Read the model definition and answer for the solid it produces. Units are mm, in the model's axes. Face numbers are marked on the shaded views. A direction names the side the tool comes from. Coordinates: 2 decimals unless noted, no trailing zeros. Order: outer loops, then holes, each group sorted by start corner. A loop starts at its lowest first (then second) coordinate and runs counter-clockwise, first axis right, second up. Notation, with made-up numbers: (64, -34.5) -> (109, -34.5) arc R32 ccw to (109, -1.5) -> close; hole circle Ø11 at (-16.5, -32.75). An arc over 180 degrees is marked (long way). Answer as a JSON object with one key per item and string values. Group by question number.
1) Section C-C on y = 135 is taken. Determine the outline of the cut face in (x, z), and give its area (3 significant figures).
2) Section D-D on x = 12.5 is taken. Determine the outline of the cut face in (y, z).
3) Section A-A on y = 45 is taken. Determine the outline of the cut face in (x, z).
4) Consider L1, parallel to Y at x = 26.75, z = 0; L2, parallel to Y at x = 28.5, z = 0.5; L3, parallel to X at y = -1.5, z = -9. Determine where each line is inside the solid, lowest interval first.
5) Given pin 1 (4 mm diameter, centred on x = 23.5, z = -6, fed in from +Y); pin 2 (5 mm diameter, centred on x = 18.5, y = 40, fed in from -Z); pin 3 (3 mm diameter, centred on x = 23, z = 4.5, fed in from +Y), each flat-ended and moving along its own axis, determine where each tip first touches the part or whether it passes through.
6) Section B-B on x = 31 is taken. Determine the outline of the cut face in (y, z), and give its area (3 significant figures).
7) Determine the mould class of the marked faces 1, 2, 3 and 4 for opening direction Z: released by +Z, released by -Z, zero draft, split by the parting line, or undercut.
8) A tool of negligible diameter and unlimited length cuts with its end or side. For the marked faces 5, 6 and 7, from which of +Z, -Z, +X, -X, +Y, -Y can it reach the whole face along a straight path? Write none if from no direction.
from build123d import *

# Parameters (mm, degrees)
SKETCH1_R               = 2
BOSS_EXTRUDE1_DEPTH     = 33
CUT_EXTRUDE1_DEPTH      = 13.5
CUT_EXTRUDE2_DEPTH      = 16.5
SKETCH4_R               = 2
CUT_EXTRUDE3_DEPTH      = 5
CUT_EXTRUDE4_DEPTH      = 3
CUT_EXTRUDE5_DEPTH      = 151.15655797
CUT_EXTRUDE5_DEPTH_BACK = 151.15655797


with BuildPart() as part:
    # Sketch1 → Boss-Extrude1 (new body)
    with BuildSketch(Plane(origin=(0, 0, 0), x_dir=(0, 0, -1), z_dir=(1, 0, 0))):
        with BuildLine():
            ThreePointArc((-15.746923292, -2.834502924), (3.806207647, -15.54068156), (15.274538651, 4.763241437))
            ThreePointArc((15.274538651, 4.763241437), (4.169990688, 68.449264041), (9.766892503, 132.853418803))
            ThreePointArc((9.766892503, 132.853418803), (2.382772527, 144.71197174), (-9.651340082, 137.617562724))
            ThreePointArc((-9.651340082, 137.617562724), (-20.507516508, 67.730411775), (-15.746923292, -2.834502924))
        make_face()
        with Locations((0, 135)):
            Circle(SKETCH1_R, mode=Mode.SUBTRACT)
        Circle(SKETCH1_R, mode=Mode.SUBTRACT)
        with BuildLine():
            ThreePointArc((-12.675406771, 58.150621112), (-12.300365948, 46.179147672), (-11.058070356, 34.266400985))
            ThreePointArc((-11.058070356, 34.266400985), (-5.587650283, 30.149080215), (-1.470329513, 35.619500288))
            ThreePointArc((-1.470329513, 35.619500288), (-2.639739364, 46.833323654), (-2.992776465, 58.102428263))
            ThreePointArc((-2.992776465, 58.102428263), (-7.809995194, 62.967839841), (-12.675406771, 58.150621112))
        make_face(mode=Mode.SUBTRACT)
        with BuildLine():
            ThreePointArc((-10.574940666, 104.538451831), (-12.44695641, 91.799336957), (-12.717862815, 78.926260385))
            ThreePointArc((-12.717862815, 78.926260385), (-7.68030208, 74.289364014), (-3.04340571, 79.326924749))
            ThreePointArc((-3.04340571, 79.326924749), (-2.79792055, 90.992020929), (-1.101570529, 102.535726074))
            ThreePointArc((-1.101570529, 102.535726074), (-4.836892719, 108.273774021), (-10.574940666, 104.538451831))
        make_face(mode=Mode.SUBTRACT)
    extrude(amount=BOSS_EXTRUDE1_DEPTH)

    # Sketch2 → Cut-Extrude1 (cut)
    with BuildSketch(Plane.ZY.offset(-8.25)):
        with BuildLine():
            ThreePointArc((9.651340082, 137.617562724), (-2.382772527, 144.71197174), (-9.766892503, 132.853418803))
            ThreePointArc((-9.766892503, 132.853418803), (-8.074404211, 124.471332441), (-6.669573364, 116.036266424))
            ThreePointArc((-6.669573364, 116.036266424), (4.209591857, 115.639688485), (13.684813674, 121.000069207))
            ThreePointArc((13.684813674, 121.000069207), (11.779096359, 129.335763119), (9.651340082, 137.617562724))
        make_face()
    extrude(amount=-CUT_EXTRUDE1_DEPTH, mode=Mode.SUBTRACT)

    # Sketch3 → Cut-Extrude2 (cut)
    with BuildSketch(Plane.ZY.offset(-8.25)):
        with BuildLine():
            ThreePointArc((15.746923292, -2.834502924), (16.932948663, 4.203707123), (17.961705011, 11.266618507))
            ThreePointArc((17.961705011, 11.266618507), (4.818924594, 21.467521501), (-11.493429399, 18.196710256))
            ThreePointArc((-11.493429399, 18.196710256), (-13.290230642, 11.453587146), (-15.274538651, 4.763241437))
            ThreePointArc((-15.274538651, 4.763241437), (-3.806207647, -15.54068156), (15.746923292, -2.834502924))
        make_face()
    extrude(amount=-CUT_EXTRUDE2_DEPTH, mode=Mode.SUBTRACT)

    # Sketch4 → Cut-Extrude3 (cut)
    with BuildSketch(Plane.ZY):
        with BuildLine():
            Line((5.508484382, 3.419742698), (6.214100211, 16.883694767))
            ThreePointArc((6.214100211, 16.883694767), (4.158233816, 19.562952015), (1.190354311, 17.951524922))
            Line((1.190354311, 17.951524922), (-3.641316221, 5.364592854))
            ThreePointArc((-3.641316221, 5.364592854), (-3.710000961, 5.241267271), (-3.810417562, 5.14205387))
            ThreePointArc((-3.810417562, 5.14205387), (-1.330634821, -6.260144645), (5.572451385, 3.147663508))
            ThreePointArc((5.572451385, 3.147663508), (5.521069981, 3.279142571), (5.508484382, 3.419742698))
        make_face()
        Circle(SKETCH4_R, mode=Mode.SUBTRACT)
    extrude(amount=-CUT_EXTRUDE3_DEPTH, mode=Mode.SUBTRACT)

    # Sketch6 → Cut-Extrude4 (cut)
    with BuildSketch(Plane.ZY.offset(-21.75)):
        with BuildLine():
            ThreePointArc((-6.669573364, 116.036266424), (-7.677372534, 122.259874843), (-8.841790135, 128.456090831))
            ThreePointArc((-8.841790135, 128.456090831), (2.534260756, 124.295910948), (10.837329247, 133.115246758))
            ThreePointArc((10.837329247, 133.115246758), (12.319974341, 127.07150219), (13.684813674, 121.000069207))
            ThreePointArc((13.684813674, 121.000069207), (4.209591857, 115.639688485), (-6.669573364, 116.036266424))
        make_face()
    extrude(amount=-CUT_EXTRUDE4_DEPTH, mode=Mode.SUBTRACT)

    # Sketch8 → Cut-Extrude5 (cut, two sides: drawn at the far end of the back side and taken through both)
    with BuildSketch(Plane.XY.offset(-CUT_EXTRUDE5_DEPTH_BACK)):
        Polygon((0, 115.000069207), (0, 25), (10, 42.320508076), (10, 97.679561131), align=None)
    extrude(amount=CUT_EXTRUDE5_DEPTH + CUT_EXTRUDE5_DEPTH_BACK, mode=Mode.SUBTRACT)


solid = part.part
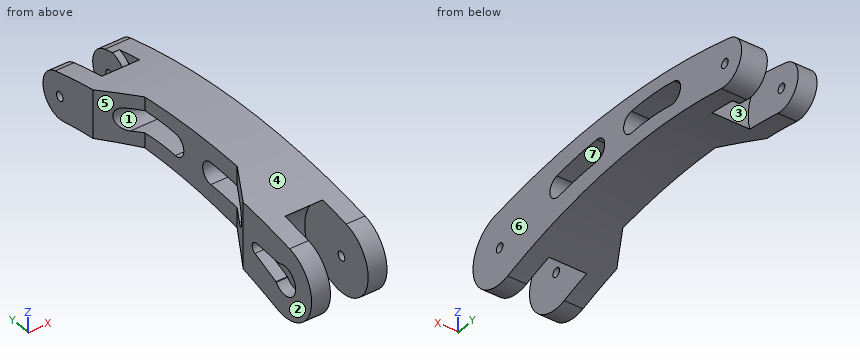
Worked answers:
{
 "1": {"outline": "(0, -10) -> (8.25, -10) -> (8.25, -2) -> (0, -2) -> close; (0, 2) -> (8.25, 2) -> (8.25, 10.35) -> (0, 10.35) -> close; (21.75, -10) -> (33, -10) -> (33, -2) -> (21.75, -2) -> close; (21.75, 2) -> (33, 2) -> (33, 10.35) -> (21.75, 10.35) -> close", "area": "319 mm²"},
 "2": {"outline": "(11.27, 17.96) arc R20 cw to (18.2, -11.49) arc R250 cw to (116.04, -6.67) arc R20 cw to (121, 13.68) arc R320 ccw to start; hole (34.27, 11.06) arc R4.84 ccw to (35.62, 1.47) arc R155.35 cw to (58.1, 2.99) arc R4.84 ccw to (58.15, 12.68) arc R165.04 ccw to start; hole (78.93, 12.72) arc R4.84 ccw to (79.33, 3.04) arc R93.5 cw to (102.54, 1.1) arc R4.84 ccw to (104.54, 10.57) arc R103.19 ccw to start"},
 "3": {"outline": "(10, -6.29) -> (33, -6.29) -> (33, 2.5) -> (10, 2.5) -> close; (10, 12.22) -> (33, 12.22) -> (33, 20.69) -> (10, 20.69) -> close"},
 "4": {"L1": "y = -16 to -2, 2 to 133, 137 to 145", "L2": "y = -15.99 to -1.94, 1.94 to 133.06, 136.94 to 144.99", "L3": "x = 0 to 8.25, 24.75 to 33"},
 "5": {"pin 1": "stops at y = 144.17", "pin 2": "stops at z = -7.44", "pin 3": "stops at y = 144.54"},
 "6": {"outline": "(-2.83, 15.75) arc R16 ccw (long way) to (4.76, -15.27) arc R250 cw to (132.85, -9.77) arc R10 ccw to (137.62, 9.65) arc R320 ccw to start; hole circle Ø4 at (0, 0); hole (34.27, 11.06) arc R4.84 ccw to (35.62, 1.47) arc R155.35 cw to (58.1, 2.99) arc R4.84 ccw to (58.15, 12.68) arc R165.04 ccw to start; hole (78.93, 12.72) arc R4.84 ccw to (79.33, 3.04) arc R93.5 cw to (102.54, 1.1) arc R4.84 ccw to (104.54, 10.57) arc R103.19 ccw to start; hole circle Ø4 at (135, 0)", "area": "3,350 mm²"},
 "7": {"face 1": "undercut", "face 2": "zero draft", "face 3": "undercut", "face 4": "released by +Z"},
 "8": {"face 5": "+Z, -Z, -X", "face 6": "+Z, -Z, +X, +Y, -Y", "face 7": "+X, -X"}
}
